from build123d import *

# Parameters (mm, degrees)
F0_W     = 130
F0_H     = 750
F1_DEPTH = 20
F2_W     = 8
F2_H     = 750
F3_DEPTH = 8
F4_W     = 8
F4_H     = 1460
F5_DEPTH = 12
F6_W     = 8
F6_H     = 750
F7_DEPTH = 12
F8_W     = 10
F8_H     = 20
F9_DEPTH = 130


with BuildPart() as f1:
    # F0 (on Front) → F1 (new body)
    with BuildSketch(Plane.XZ):
        with Locations((-309.722924, 109.476302)):
            Rectangle(F0_W, F0_H)
    extrude(amount=-F1_DEPTH)

    # F2 (on face) → F3 (cut)
    with BuildSketch(Plane.XZ):
        with Locations((-309.722924, 109.476302)):
            Rectangle(F2_W, F2_H)
    extrude(amount=-F3_DEPTH, mode=Mode.SUBTRACT)

    # F4 (on face) → F5 (cut)
    with BuildSketch(Plane.XZ):
        with Locations((-370.722924, -245.523698)):
            Rectangle(F4_W, F4_H)
    extrude(amount=-F5_DEPTH, mode=Mode.SUBTRACT)

    # F6 (on face) → F7 (cut)
    with BuildSketch(Plane(origin=(0, 20, 0), x_dir=(-1, 0, 0), z_dir=(0, 1, 0))):
        with Locations((248.722924, 109.476302)):
            Rectangle(F6_W, F6_H)
    extrude(amount=-F7_DEPTH, mode=Mode.SUBTRACT)

    # F8 (on face) → F9 (cut)
    with BuildSketch(Plane(origin=(-366.722924, 0, 0), x_dir=(0, -1, 0), z_dir=(-1, 0, 0))):
        with Locations((-5, -205.523698)):
            Rectangle(F8_W, F8_H)
        with Locations((-5, 424.476302)):
            Rectangle(F8_W, F8_H)
    extrude(amount=-F9_DEPTH, mode=Mode.SUBTRACT)


solid = f1.part
Check sheet for the modelled part. Datum: model origin and axes. Units: mm. A direction names the side the tool comes from. Give positions to 0.01 mm unless a question says otherwise; leave off trailing zeros. Write each loop counter-clockwise with the first axis right and the second up, starting at its lowest first coordinate (ties: lowest second). Pieces come first, ordered by that corner, then holes. Notation, with made-up numbers: (12.25, 10.25) -> (58.25, 10.25) arc R31 ccw to (58.25, 36.25) -> close; hole circle Ø2 at (48, -6.5). An arc over 180 degrees is marked (long way). One line per item, written item: value. Start each with the question number.
Item 1: Section check C-C on y = 16.25. Record the cut outline in (x, z).
Item 2: Section check B-B on x = -354. Record the cut outline in (y, z).
Item 3: Tool access check on faces 1 (the flat face through (-276, 0, 460)), 2 (the flat face through (-311, 10, -206)), 3 (the flat face through (-366.723, 6, 104)), 4 (the flat face through (-315, 20, 115)), 5 (the flat face through (-252.723, 14, 104)). Record the directions out of +Z, -Z, +X, -X, +Y, -Y that give a thin tool (end or side, any length) a straight path to the whole face; none if there is none.
Item 4: Material ranges on probe 1 along Z at (x, y) = (-364.5, 5.75); probe 2 along X at (y, z) = (3, -191.5); probe 3 along X at (y, z) = (18, -134), recorded low to high. Write a range as from..to.
Item 5: Section check A-A on z = 205.5. Record the cut outline in (x, y), then the cut area to 3 significant figures.
Item 6: Gauge pin test, flat ends, axial feed: pin 1 (3 mm diameter, centred on x = -306, y = 4.5, fed in from +Z); pin 2 (5 mm diameter, centred on y = 17, z = 246, fed in from +X); pin 3 (4 mm diameter, centred on y = 2.5, z = 262, fed in from -X); pin 4 (2.5 mm diameter, centred on x = -248, z = 56.5, fed in from +Y). Record the tip position at first contact, or that the pin passes through.
Results list:
1. outline: (-374.72, -265.52) -> (-252.72, -265.52) -> (-252.72, 484.48) -> (-374.72, 484.48) -> close
2. outline: (0, -265.52) -> (20, -265.52) -> (20, 484.48) -> (0, 484.48) -> (0, 434.48) -> (10, 434.48) -> (10, 414.48) -> (0, 414.48) -> (0, -195.52) -> (10, -195.52) -> (10, -215.52) -> (0, -215.52) -> close
3. face 1: +Z, -Z, +X, -X, -Y
3. face 2: +X, -X, -Y
3. face 3: +Z, -Z, -X, -Y
3. face 4: +Z, -Z, +X, -X, +Y
3. face 5: +Z, -Z, +X, +Y
4. probe 1: -265.52..-215.52, -195.52..414.48, 434.48..484.48
4. probe 2: -366.72..-313.72, -305.72..-244.72
4. probe 3: -374.72..-252.72
5. outline: (-374.72, 12) -> (-366.72, 12) -> (-366.72, 0) -> (-313.72, 0) -> (-313.72, 8) -> (-305.72, 8) -> (-305.72, 0) -> (-244.72, 0) -> (-244.72, 8) -> (-252.72, 8) -> (-252.72, 20) -> (-374.72, 20) -> close
5. area: 2,340 mm²
6. pin 1: z = 484.48
6. pin 2: x = -252.72
6. pin 3: x = -366.72
6. pin 4: y = 8
